Geometry check sheet. Reference: the model listing, model coordinates, mm. Coordinates: 2 decimals unless noted, no trailing zeros. One line per item, written item: value. Start each with the question number.
1) Thickness scan on L1, parallel to Z at x = 415.5, y = 11.6; L2, parallel to Z at x = 357.5, y = 10.75; L3, parallel to X at y = 0, z = 4.75. Record the ranges inside material, lowest first. Write a range as from..to.
2) Sectioned sample at A-A, the plane x = -122.5. State how many separate pieces and enclosed holes the cut face has, then the cut area to 3 significant figures.
3) Go/stop test with flat-tipped pins: P1, Ø6, axis at x = -32, z = 0, coming from the -Y side; P2, Ø6, axis at x = -78.73, y = 0, coming from the +Z side; P3, Ø1.5, axis at y = -7.5, z = -2.5, coming from the +X side; P4, Ø2, axis at x = 485, y = 1, coming from the -Z side. Record where each tip stops, or that it passes through.
```python
from build123d import *

# Parameters (mm, degrees)
SKETCH11_R                = 3.4
SKETCH11_R_2              = 2
NEW_ALUM_ALUM3BY3_1_DEPTH = 1050
SKETCH12_R                = 2.5
CUT_EXTRUDE1_DEPTH        = 707.780320658


with BuildPart() as part:
    # Sketch11 → New alum ALUM3BY3(1) (new body)
    with BuildSketch(Plane.YZ.offset(-343.690987124)):
        with BuildLine():
            Line((-4, 6), (4, 6))
            Line((4, 6), (8.25, 10.106126974))
            Line((8.25, 10.106126974), (8.25, 13))
            Line((8.25, 13), (4, 13))
            Line((4, 13), (4, 15))
            Line((4, 15), (13, 15))
            ThreePointArc((13, 15), (14.414213562, 14.414213562), (15, 13))
            Line((15, 13), (15, 4))
            Line((15, 4), (13, 4))
            Line((13, 4), (13, 8.25))
            Line((13, 8.25), (10.398914138, 8.25))
            Line((10.398914138, 8.25), (6, 4))
            Line((6, 4), (6, -4))
            Line((6, -4), (10.398914138, -8.25))
            Line((10.398914138, -8.25), (13, -8.25))
            Line((13, -8.25), (13, -4))
            Line((13, -4), (15, -4))
            Line((15, -4), (15, -13))
            ThreePointArc((15, -13), (14.414213562, -14.414213562), (13, -15))
            Line((13, -15), (4, -15))
            Line((4, -15), (4, -13))
            Line((4, -13), (8.25, -13))
            Line((8.25, -13), (8.25, -10.106126974))
            Line((8.25, -10.106126974), (4, -6))
            Line((4, -6), (-4, -6))
            Line((-4, -6), (-8.25, -10.106126974))
            Line((-8.25, -10.106126974), (-8.25, -13))
            Line((-8.25, -13), (-4, -13))
            Line((-4, -13), (-4, -15))
            Line((-4, -15), (-13, -15))
            ThreePointArc((-13, -15), (-14.414213562, -14.414213562), (-15, -13))
            Line((-15, -13), (-15, -4))
            Line((-15, -4), (-13, -4))
            Line((-13, -4), (-13, -8.25))
            Line((-13, -8.25), (-10.398914138, -8.25))
            Line((-10.398914138, -8.25), (-6, -4))
            Line((-6, -4), (-6, 4))
            Line((-6, 4), (-10.398914138, 8.25))
            Line((-10.398914138, 8.25), (-13, 8.25))
            Line((-13, 8.25), (-13, 4))
            Line((-13, 4), (-15, 4))
            Line((-15, 4), (-15, 13))
            ThreePointArc((-15, 13), (-14.414213562, 14.414213562), (-13, 15))
            Line((-13, 15), (-4, 15))
            Line((-4, 15), (-4, 13))
            Line((-4, 13), (-8.25, 13))
            Line((-8.25, 13), (-8.25, 10.106126974))
            Line((-8.25, 10.106126974), (-4, 6))
        make_face()
        Circle(SKETCH11_R, mode=Mode.SUBTRACT)
        with Locations((11.6, 11.6)):
            Circle(SKETCH11_R_2, mode=Mode.SUBTRACT)
        with Locations((-11.6, 11.6)):
            Circle(SKETCH11_R_2, mode=Mode.SUBTRACT)
        with Locations((11.6, -11.6)):
            Circle(SKETCH11_R_2, mode=Mode.SUBTRACT)
        with Locations((-11.6, -11.6)):
            Circle(SKETCH11_R_2, mode=Mode.SUBTRACT)
    extrude(amount=NEW_ALUM_ALUM3BY3_1_DEPTH)

    # Sketch12 → Cut-Extrude1 (cut, through all)
    with BuildSketch(Plane.XY.offset(6)):
        with Locations((-268.690987124, 0)):
            Circle(SKETCH12_R)
        with Locations((-168.690987124, 0)):
            Circle(SKETCH12_R)
        with Locations((-78.730987124, 0)):
            Circle(SKETCH12_R)
    extrude(amount=-CUT_EXTRUDE1_DEPTH, mode=Mode.SUBTRACT)


solid = part.part
```
Final values:
1. L1: z = -15..-13.6, -9.6..-8.25, 8.25..9.6, 13.6..15
1. L2: z = -15..-13.41, -9.79..-8.25, 8.25..9.79, 13.41..15
1. L3: x = -343.69..-271.19, -266.19..-171.19, -166.19..-81.23, -76.23..706.31
2. separate pieces: 1
2. enclosed holes: 5
2. area: 356 mm^2
3. P1: stops at y = -6
3. P2: stops at z = 6
3. P3: passes through
3. P4: stops at z = -6
